Work out the finished part from the listing and answer in its coordinate system (mm). Coordinates: 2 decimals unless noted, no trailing zeros. Write each loop counter-clockwise with the first axis right and the second up, starting at its lowest first coordinate (ties: lowest second). Pieces come first, ordered by that corner, then holes. Notation, with made-up numbers: M -37,15 L -28,15 A22 ccw -28,40 Z; hole C 74.25,21 d5. An arc over 180 degrees is marked long. Use CSV: the item, a comma, the result in double quotes.
Autodesk Inventor part; units mm, degrees
ref_plane "YZ Plane" through (0, 0, 0) normal (1, 0, 0) x (0, 1, 0)
ref_plane "XZ Plane" through (0, 0, 0) normal (0, 1, 0) x (-1, 0, 0)
ref_plane "XY Plane" through (0, 0, 0) normal (0, 0, 1) x (1, 0, 0)
sketch "Sketch1" plane through (0, 0, 0) normal (0, 0, 1) x (1, 0, 0)
  line L0 (0, 0) -> (145.2, 0)
  line L1 (145.2, 0) -> (145.2, 192)
  line L2 (145.2, 192) -> (0, 192)
  line L3 (0, 192) -> (0, 0)
  line L4 (145.2, 192) -> (110.498, 192)
  line L5 (145.2, 186.8) -> (145.2, 192)
  line L6 (85.92, 192) -> (45.5217, 192)
  line L7 (21.953, 192) -> (0, 192)
  line L8 (0, 192) -> (0, 185.7065)
  line L9 (35.2, 192) -> (60.2, 192)
  line L10 (60.2, 192) -> (60.2, 186.8)
  line L11 (60.2, 186.8) -> (35.2, 186.8)
  line L12 (35.2, 186.8) -> (35.2, 192)
  line L13 (90.2, 192) -> (115.2, 192)
  line L14 (115.2, 192) -> (115.2, 186.8)
  line L15 (115.2, 186.8) -> (90.2, 186.8)
  line L16 (90.2, 186.8) -> (90.2, 192)
  line L17 (0, 192) -> (5.2, 192)
  line L18 (5.2, 192) -> (5.2, 142)
  line L19 (5.2, 142) -> (0, 142)
  line L20 (0, 142) -> (0, 192)
  line L21 (0, 96) -> (145.2, 96) construction
  line L22 (0, 0) -> (5.2, 0)
  line L23 (5.2, 0) -> (5.2, 50)
  line L24 (5.2, 50) -> (0, 50)
  line L25 (0, 50) -> (0, 0)
  line L26 (35.2, 0) -> (60.2, 0)
  line L27 (60.2, 0) -> (60.2, 5.2)
  line L28 (60.2, 5.2) -> (35.2, 5.2)
  line L29 (35.2, 5.2) -> (35.2, 0)
  line L30 (90.2, 0) -> (115.2, 0)
  line L31 (115.2, 0) -> (115.2, 5.2)
  line L32 (115.2, 5.2) -> (90.2, 5.2)
  line L33 (90.2, 5.2) -> (90.2, 0)
  circle A0 centre (102, 96) radius 2.5
  circle A1 centre (27, 96) radius 11.5
  circle A2 centre (42.5, 80.5) radius 1.5
  circle A3 centre (42.5, 111.5) radius 1.5
  circle A4 centre (11.5, 111.5) radius 1.5
  circle A5 centre (11.5, 80.5) radius 1.5
  dimension "d0" = 192
  dimension "d1" = 145.2
  dimension "d6" = 25
  dimension "d7" = 25
  dimension "d8" = 5.2
  dimension "d9" = 30
  dimension "d10" = 30
  dimension "d11" = 50
  dimension "d12" = 5.2
  dimension "d13" = 50
  dimension "d14" = 5.2
  dimension "d15" = 25
  dimension "d16" = 25
  dimension "d17" = 5.2
  dimension "d18" = 30
  dimension "d19" = 30
  dimension "d22" = 5
  dimension "d24" = 23
  dimension "d25" = 3
  dimension "d26" = 15.5
  dimension "d27" = 15.5
  dimension "d30" = 360
  dimension "d32" = 75
  dimension "d33" = 27
extrude "Extrusion2" add sketch "Sketch1" along normal blind 5.2 contours L23 L24 L3 L19 L18 L2 L12 L11 L10 L16 L15 L14 L1 L0 L31 L32 L33 L27 L28 L29
properties part number "Base Plate"
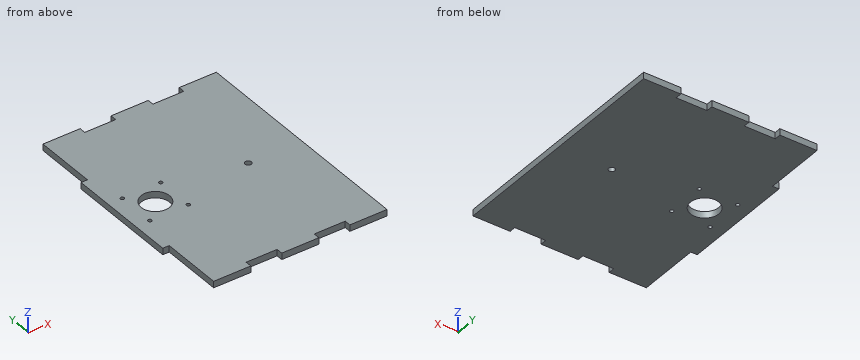
Item 1: Consider probe 1 along X at (y, z) = (80.5, 2.75); probe 2 along Y at (x, z) = (11.5, 1.75); probe 3 along Y at (x, z) = (42.5, 1.4). Determine where each line is inside the solid, lowest interval first.
Answer:
probe 1,"x = 0 to 10, 13 to 41, 44 to 145.2"
probe 2,"y = 0 to 79, 82 to 110, 113 to 192"
probe 3,"y = 5.2 to 79, 82 to 110, 113 to 186.8"
Item 2: The part is cut by section C-C (z = 1.55). Count the separate pieces of the cut face and the enclosed holes in it, then the cut area to 3 significant figures.
Answer:
separate pieces,"1"
enclosed holes,"6"
area,"26,400 mm2"
Item 3: The part is cut by section B-B (y = 96). Write down the section's boundary in (x, z).
Answer:
outline,"M 0,0 L 15.5,0 L 15.5,5.2 L 0,5.2 Z; M 38.5,0 L 99.5,0 L 99.5,5.2 L 38.5,5.2 Z; M 104.5,0 L 145.2,0 L 145.2,5.2 L 104.5,5.2 Z"
Item 4: The part is cut by section D-D (y = 164.5). Write down the section's boundary in (x, z), then the cut area to 3 significant figures.
Answer:
outline,"M 5.2,0 L 145.2,0 L 145.2,5.2 L 5.2,5.2 Z"
area,"728 mm2"
Item 5: The part is cut by section A-A (x = 27). Write down the section's boundary in (y, z).
Answer:
outline,"M 0,0 L 84.5,0 L 84.5,5.2 L 0,5.2 Z; M 107.5,0 L 192,0 L 192,5.2 L 107.5,5.2 Z"
Item 6: Given pin 1 (1 mm diameter, centred on y = 162, z = 2.5, fed in from -X); pin 2 (2.5 mm diameter, centred on x = 44, z = 3, fed in from -Y); pin 3 (2.5 mm diameter, centred on x = 44.5, z = 3.5, fed in from +Y), each flat-ended and moving along its own axis, determine where each tip first touches the part or whether it passes through.
Answer:
pin 1,"stops at x = 5.2"
pin 2,"stops at y = 5.2"
pin 3,"stops at y = 186.8"
